The model under review builds one solid part; all positions refer to its coordinate system, in mm. A direction names the side the tool comes from. Round coordinates to 2 decimals unless told otherwise and drop trailing zeros. Write each loop counter-clockwise with the first axis right and the second up, starting at its lowest first coordinate (ties: lowest second). Pieces come first, ordered by that corner, then holes. Notation, with made-up numbers: M 83,78.5 L 88,78.5 A20 cw 88,83.5 Z; hole C 70.25,-11.75 d4. An arc over 180 degrees is marked long. One line per item, written item: value. Start each with the question number.
1) Take a section at C-C, the plane z = 17.5. State how many separate pieces and enclosed holes the cut face has, and give its area (3 significant figures).
2) Take a section at B-B, the plane z = -21.5. Write out the cut boundary in (x, y), and give its area (3 significant figures).
3) Mouldability with a two-part tool opening along X and no side actions: class faces 1 (the face through (-24, 0, 0)), 2 (the face through (30, 0, 18)), 3 (the face through (28.028, 0.225, 29.285)) as +X half, -X half, draft (parallel to the pull), parting line (faces both ways), or undercut.
4) Take a section at D-D, the plane x = -23. Write out the cut boundary in (y, z), and give its area (3 significant figures).
5) Tool access review of faces 4 (the face through (-23, -13, 0)), 5 (the face through (-28.03, 13.01, 16.95)), 6 (the face through (23, 13, 0)), 7 (the face through (26, 7, 21)): name each direction out of +Z, -Z, +X, -X, +Y, -Y from which nothing blocks a thin tool from reaching the whole face with its end or side.
6) Take a section at A-A, the plane y = 12.5. Write out the cut boundary in (x, z), and give its area (3 significant figures).
7) For P1, Ø3, axis at y = -1.5, z = -7.5, coming from the +X side; P2, Ø2.5, axis at y = 12.5, z = 17.5, coming from the +X side; P3, Ø5, axis at y = -1, z = -5.5, coming from the -X side; P4, Ø1.4, axis at y = 12.5, z = 17.5, coming from the -X side, all flat-tipped, find the tip position at first contact; note any pin that passes through.
8) Wall thickness on probe 1 along X at (y, z) = (-6.5, 8); probe 2 along X at (y, z) = (8.75, -23); probe 3 along Y at (x, z) = (-28, 17): over which ranges is each line inside the solid? List them lowest first.
from build123d import *

# Parameters (mm, degrees)
BOSS_EXTRUDE1_DEPTH = 32.5
BOSS_EXTRUDE2_START = 2
SKETCH2_R           = 15
BOSS_EXTRUDE2_DEPTH = 4
SKETCH3_R           = 7.5
BOSS_EXTRUDE3_DEPTH = 50
SKETCH4_R           = 15
BOSS_EXTRUDE4_DEPTH = 4
SKETCH5_R           = 0.75
CUT_EXTRUDE1_DEPTH  = 4
SKETCH6_R           = 0.75
CUT_EXTRUDE2_DEPTH  = 4


with BuildPart() as part:
    # Sketch1 → Boss-Extrude1 (new body, symmetric)
    with BuildSketch(Plane.XY):
        with BuildLine():
            Line((-19, -15), (19, -15))
            ThreePointArc((19, -15), (22.535533906, -13.535533906), (24, -10))
            Line((24, -10), (24, 10))
            ThreePointArc((24, 10), (22.535533906, 13.535533906), (19, 15))
            Line((19, 15), (-19, 15))
            ThreePointArc((-19, 15), (-22.535533906, 13.535533906), (-24, 10))
            Line((-24, 10), (-24, -10))
            ThreePointArc((-24, -10), (-22.535533906, -13.535533906), (-19, -15))
        make_face()
    extrude(amount=BOSS_EXTRUDE1_DEPTH, both=True)



with BuildPart() as body_2:
    # Sketch2 → Boss-Extrude2 (new body)
    with BuildSketch(Plane(origin=(24, 0, 0), x_dir=(0, 0, -1), z_dir=(1, 0, 0)).offset(BOSS_EXTRUDE2_START)):
        with Locations((-17.5, 0)):
            Circle(SKETCH2_R)
    extrude(amount=BOSS_EXTRUDE2_DEPTH)


with BuildPart() as part_1:
    add(part.part)

    add(body_2.part)  # Boss-Extrude3 merges body 2
    # Sketch3 → Boss-Extrude3 (add)
    with BuildSketch(Plane.ZY.offset(-26)):
        with Locations((17.5, 0)):
            Circle(SKETCH3_R)
    boss_extrude3 = extrude(amount=BOSS_EXTRUDE3_DEPTH)

    # Mirror3: Boss-Extrude3 across plane
    add(boss_extrude3.mirror(Plane(origin=(0, 0, 0), x_dir=(0, 0, 1), z_dir=(1, 0, 0))))

    # Sketch4 → Boss-Extrude4 (add)
    with BuildSketch(Plane.ZY.offset(26)):
        with Locations((17.5, 0)):
            Circle(SKETCH4_R)
    extrude(amount=BOSS_EXTRUDE4_DEPTH)

    # Sketch5 → Cut-Extrude1 (cut)
    with BuildSketch(Plane(origin=(30, 0, 0), x_dir=(0, 0, -1), z_dir=(1, 0, 0))):
        with Locations((-17.5, 12.5)):
            Circle(SKETCH5_R)
        with Locations((-8.661165235, 8.838834765)):
            Circle(SKETCH5_R)
        with Locations((-5, 0)):
            Circle(SKETCH5_R)
        with Locations((-8.661165235, -8.838834765)):
            Circle(SKETCH5_R)
        with Locations((-17.5, -12.5)):
            Circle(SKETCH5_R)
        with Locations((-26.338834765, -8.838834765)):
            Circle(SKETCH5_R)
        with Locations((-30, 0)):
            Circle(SKETCH5_R)
        with Locations((-26.338834765, 8.838834765)):
            Circle(SKETCH5_R)
    extrude(amount=-CUT_EXTRUDE1_DEPTH, mode=Mode.SUBTRACT)

    # Sketch6 → Cut-Extrude2 (cut)
    with BuildSketch(Plane.ZY.offset(30)):
        with Locations((17.5, 12.5)):
            Circle(SKETCH6_R)
        with Locations((26.338834765, 8.838834765)):
            Circle(SKETCH6_R)
        with Locations((30, 0)):
            Circle(SKETCH6_R)
        with Locations((26.338834765, -8.838834765)):
            Circle(SKETCH6_R)
        with Locations((17.5, -12.5)):
            Circle(SKETCH6_R)
        with Locations((8.661165235, -8.838834765)):
            Circle(SKETCH6_R)
        with Locations((5, 0)):
            Circle(SKETCH6_R)
        with Locations((8.661165235, 8.838834765)):
            Circle(SKETCH6_R)
    extrude(amount=-CUT_EXTRUDE2_DEPTH, mode=Mode.SUBTRACT)


solid = part_1.part
Checked values:
1. separate pieces: 5
1. enclosed holes: 0
1. area: 1,690 mm2
2. outline: M -24,-10 A5 ccw -19,-15 L 19,-15 A5 ccw 24,-10 L 24,10 A5 ccw 19,15 L -19,15 A5 ccw -24,10 Z
2. area: 1,420 mm2
3. face 1: undercut
3. face 2: +X half
3. face 3: draft
4. outline: M -13,-32.5 L 13,-32.5 L 13,32.5 L -13,32.5 Z
4. area: 1,690 mm2
5. face 4: +Z, -Z, -Y
5. face 5: -X
5. face 6: +Z, -Z, +Y
5. face 7: none
6. outline: M -30,9.21 L -26,9.21 L -26,16.75 L -30,16.75 Z; M -30,18.25 L -26,18.25 L -26,25.79 L -30,25.79 Z; M -23.33,-32.5 L 23.33,-32.5 L 23.33,32.5 L -23.33,32.5 Z; M 26,9.21 L 30,9.21 L 30,16.75 L 26,16.75 Z; M 26,18.25 L 30,18.25 L 30,25.79 L 26,25.79 Z
6. area: 3,150 mm2
7. P1: stops at x = 24
7. P2: stops at x = 30
7. P3: stops at x = -24
7. P4: stops at x = -23.66
8. probe 1: x = -30 to -26, -24 to 24, 26 to 30
8. probe 2: x = -24 to 24
8. probe 3: y = -14.99 to -13.06, -11.94 to 11.94, 13.06 to 14.99
